Here's how the part is built. I have some questions about the finished solid (model axes, mm). Face numbers are marked on the shaded views. A direction names the side the tool comes from. Give positions to 0.01 mm unless a question says otherwise; leave off trailing zeros. Loops run counter-clockwise (first coordinate to the right, second up) from the corner with the lowest first, then second, coordinate; pieces in that order, holes last.
Q1. If we section it at B-B (z = 8.5): Please give me the cut outline in (x, y).
Q2. We'd pull the mould along X, two halves only. Please class the marked faces 1, 2 and 3: +X half, -X half, draft (parallel to the pull), parting line (faces both ways), or undercut.
Q3. If we section it at C-C (x = 17): Please give me the cut outline in (y, z), plus the area to 3 significant figures.
Q4. If we section it at D-D (y = -20.5): Please give me the cut outline in (x, z), plus the area to 3 significant figures.
Q5. If we section it at A-A (y = -10.5): Please give me the cut outline in (x, z).
Q6. Will these pins go through, and if not, where does the flat tip stop? P1, Ø6, axis at x = 17, y = -12.5, coming from the -Z side; P2, Ø1, axis at x = 11, z = 14, coming from the +Y side; P3, Ø2, axis at y = -21, z = 18.5, coming from the +X side; P4, Ø1, axis at x = 10.5, y = -8.5, coming from the +Z side.
Q7. I need wall thicknesses on line 1 (Y direction, x = 17, z = 11.55); line 2 (X direction, y = -3.25, z = 6.5); line 3 (Z direction, x = 11.5, y = -12.75). Which ranges of each line are inside material? Lowest first, please.
Q8. For the marked faces 4, 5, 6, 7 and 8, which set-ups out of +Z, -Z, +X, -X, +Y, -Y let a thin tool reach every point of the face, with its end or its side?
from build123d import *

# Parameters (mm, degrees)
F1_DEPTH = 25
F2_R     = 2.5
F3_DEPTH = 25
F4_R     = 1
F5_DEPTH = 5


with BuildPart() as f1:
    # F0 (on Front) → F1 (new body)
    with BuildSketch(Plane.XZ):
        with BuildLine():
            Line((-3, 0), (0, 0))
            Line((0, 0), (0, 17))
            ThreePointArc((0, 17), (0.87868, 19.12132), (3, 20))
            Line((3, 20), (5, 20))
            ThreePointArc((5, 20), (7.12132, 19.12132), (8, 17))
            Line((8, 17), (8, 13))
            ThreePointArc((8, 13), (8.87868, 10.87868), (11, 10))
            Line((11, 10), (23, 10))
            Line((23, 10), (23, 13))
            Line((23, 13), (11, 13))
            Line((11, 13), (11, 17))
            ThreePointArc((11, 17), (9.242641, 21.242641), (5, 23))
            Line((5, 23), (3, 23))
            ThreePointArc((3, 23), (-1.242641, 21.242641), (-3, 17))
            Line((-3, 17), (-3, 0))
        make_face()
    extrude(amount=F1_DEPTH)

    # F2 (on face) → F3 (cut)
    with BuildSketch(Plane.XY.offset(13)):
        with Locations((17, -12.5)):
            Circle(F2_R)
        with BuildLine():
            Line((14.55051, -25), (19.44949, -25))
            ThreePointArc((19.44949, -25), (19.48734, -24.751272), (19.5, -24.5))
            ThreePointArc((19.5, -24.5), (16.748728, -22.01266), (14.55051, -25))
        make_face()
        with BuildLine():
            ThreePointArc((14.55051, 0), (16.748728, -2.98734), (19.5, -0.5))
            ThreePointArc((19.5, -0.5), (19.48734, -0.248728), (19.44949, 0))
            Line((19.44949, 0), (14.55051, 0))
        make_face()
    extrude(amount=-F3_DEPTH, mode=Mode.SUBTRACT)

    # F4 (on face) → F5 (cut)
    with BuildSketch(Plane(origin=(-3, 0, 0), x_dir=(0, -1, 0), z_dir=(-1, 0, 0))):
        with Locations((18.75, 8.5)):
            Circle(F4_R)
        with Locations((6.25, 8.5)):
            Circle(F4_R)
    extrude(amount=-F5_DEPTH, mode=Mode.SUBTRACT)


solid = f1.part
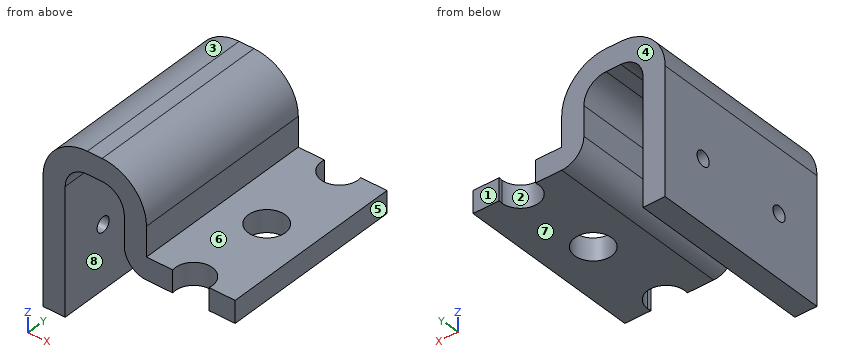
Check sheet entries:
1. outline: (-3, -25) - (0, -25) - (0, -19.75) - (-3, -19.75) - close; (-3, -17.75) - (0, -17.75) - (0, -7.25) - (-3, -7.25) - close; (-3, -5.25) - (0, -5.25) - (0, 0) - (-3, 0) - close
2. face 1: draft
2. face 2: undercut
2. face 3: -X half
3. outline: (-22, 10) - (-15, 10) - (-15, 13) - (-22, 13) - close; (-10, 10) - (-3, 10) - (-3, 13) - (-10, 13) - close
3. area: 42.0 mm2
4. outline: (-3, 0) - (0, 0) - (0, 17) arc R3 cw to (3, 20) - (5, 20) arc R3 cw to (8, 17) - (8, 13) arc R3 ccw to (11, 10) - (23, 10) - (23, 13) - (11, 13) - (11, 17) arc R6 ccw to (5, 23) - (3, 23) arc R6 ccw to (-3, 17) - close
4. area: 154 mm2
5. outline: (-3, 0) - (0, 0) - (0, 17) arc R3 cw to (3, 20) - (5, 20) arc R3 cw to (8, 17) - (8, 13) arc R3 ccw to (11, 10) - (15.5, 10) - (15.5, 13) - (11, 13) - (11, 17) arc R6 ccw to (5, 23) - (3, 23) arc R6 ccw to (-3, 17) - close; (18.5, 10) - (23, 10) - (23, 13) - (18.5, 13) - close
6. P1: stops at z = 10
6. P2: stops at y = 0
6. P3: stops at x = 10.98
6. P4: stops at z = 20.32
7. line 1: y = -22 to -15, -10 to -3
7. line 2: x = -3 to 0
7. line 3: z = 10 to 13
8. face 4: +Z, -Z, +X, -X, +Y
8. face 5: +Z, -Z, +X, +Y, -Y
8. face 6: +Z, +X, +Y, -Y
8. face 7: -Z, +X, +Y, -Y
8. face 8: -Z, +Y, -Y
